Read the model definition and answer for the solid it produces. Units are mm, in the model's axes. A direction names the side the tool comes from. Round coordinates to 2 decimals unless told otherwise and drop trailing zeros. Write each loop counter-clockwise with the first axis right and the second up, starting at its lowest first coordinate (ties: lowest second). Pieces come first, ordered by that corner, then holes. Notation, with made-up numbers: (-39.5, 57) -> (-27.5, 57) arc R19 cw to (-27.5, 65) -> close; hole circle Ø2 at (53, -14.5). An arc over 180 degrees is marked (long way). Return JSON: item names as keys, results as strings.
from build123d import *

# Parameters (mm, degrees)
SKETCH1_R           = 9
SKETCH1_R_2         = 2.75
SKETCH1_R_3         = 2.5
BOSS_EXTRUDE1_DEPTH = 3
SKETCH4_R           = 5
SKETCH4_W           = 3
SKETCH4_H           = 5
BOSS_EXTRUDE4_DEPTH = 10


with BuildPart() as part:
    # Sketch1 → Boss-Extrude1 (new body)
    with BuildSketch(Plane(origin=(0, 0, 0), x_dir=(1, 0, 0), z_dir=(0, 1, 0))):
        Circle(SKETCH1_R)
        with Locations((-5, 0.000835232)):
            Circle(SKETCH1_R_2, mode=Mode.SUBTRACT)
        with Locations((5, 0)):
            Circle(SKETCH1_R_3, mode=Mode.SUBTRACT)
    extrude(amount=BOSS_EXTRUDE1_DEPTH)

    # Sketch4 → Boss-Extrude4 (add)
    with BuildSketch(Plane(origin=(0, 3, 0), x_dir=(1, 0, 0), z_dir=(0, 1, 0))):
        with Locations((1.5, 0)):
            Circle(SKETCH4_R)
        Rectangle(SKETCH4_W, SKETCH4_H, mode=Mode.SUBTRACT)
    extrude(amount=BOSS_EXTRUDE4_DEPTH)


solid = part.part
Item 1: For a pull along Z with two mould halves and no side action, classify faces 1 (the cylindrical face through (-1.172, 1.479, -8.923)), 2 (the cylindrical face through (7.385, 1.479, -0.751)), 3 (the flat face through (3, 13, 0)) as released by +Z, released by -Z, zero draft, split by the parting line, or undercut.
Worked answers:
{"face 1": "split by the parting line", "face 2": "undercut", "face 3": "zero draft"}
Item 2: Straight lines are drawn through the part: L1, parallel to X at y = 2.1, z = 0; L2, parallel to X at y = 2.5, z = -0.5; L3, parallel to X at y = 3.25, z = -0.25. For each, find the intervals that lie inside material, in ascending order. Write a range as [from, to].
Worked answers:
{"L1": "x = [-9, -7.75], [-2.25, 2.5], [7.5, 9]", "L2": "x = [-8.99, -7.7], [-2.3, 2.55], [7.45, 8.99]", "L3": "x = [-3.49, -1.5], [1.5, 6.49]"}
Item 3: Section C-C (z = -0.75) is taken. Give the vertices of the cut face in (x, y), then the cut area to 3 significant figures.
Worked answers:
{"outline": "(-8.97, 0) -> (-7.65, 0) -> (-7.65, 3) -> (-8.97, 3) -> close; (-3.44, 3) -> (-2.35, 3) -> (-2.35, 0) -> (2.62, 0) -> (2.62, 3) -> (6.44, 3) -> (6.44, 13) -> (1.5, 13) -> (1.5, 3) -> (-1.5, 3) -> (-1.5, 13) -> (-3.44, 13) -> close; (7.38, 0) -> (8.97, 0) -> (8.97, 3) -> (7.38, 3) -> close", "area": "92.5 mm2"}
Item 4: Section B-B (y = 6.25) is taken. Give the vertices of the cut face in (x, z).
Worked answers:
{"outline": "circle Ø10 at (1.5, 0); hole (-1.5, -2.5) -> (1.5, -2.5) -> (1.5, 2.5) -> (-1.5, 2.5) -> close"}
Item 5: Flat-ended cylindrical pins translate along their axes: pin 1 (3.5 mm diameter, centred on x = 0.5, y = 7, fed in from -Z); pin 2 (4 mm diameter, centred on y = 6.5, z = 0, fed in from +X); pin 3 (1.2 mm diameter, centred on x = 3.5, z = -1, fed in from -Y). Find the tip coordinate at first contact, or state that the pin passes through.
Worked answers:
{"pin 1": "stops at z = -5", "pin 2": "stops at x = 6.5", "pin 3": "stops at y = 3"}
Item 6: Section A-A (x = -5) is taken. Give the vertices of the cut face in (y, z).
Worked answers:
{"outline": "(0, -7.48) -> (3, -7.48) -> (3, -2.75) -> (0, -2.75) -> close; (0, 2.75) -> (3, 2.75) -> (3, 7.48) -> (0, 7.48) -> close"}
Item 7: Section D-D (x = 2) is taken. Give the vertices of the cut face in (y, z).
Worked answers:
{"outline": "(0, -8.77) -> (3, -8.77) -> (3, -4.97) -> (13, -4.97) -> (13, 4.97) -> (3, 4.97) -> (3, 8.77) -> (0, 8.77) -> close"}
Item 8: A tool of negligible diameter and unlimited length cuts with its end or side. For faces 4 (the flat face through (0, 8, -2.5)), 5 (the flat face through (4, 3, 0)), 6 (the flat face through (0, 0, 0)), from which of +Z, -Z, +X, -X, +Y, -Y can it reach the whole face along a straight path? Write none if from no direction.
Worked answers:
{"face 4": "+Y", "face 5": "-Y", "face 6": "+Z, -Z, +X, -X, -Y"}
